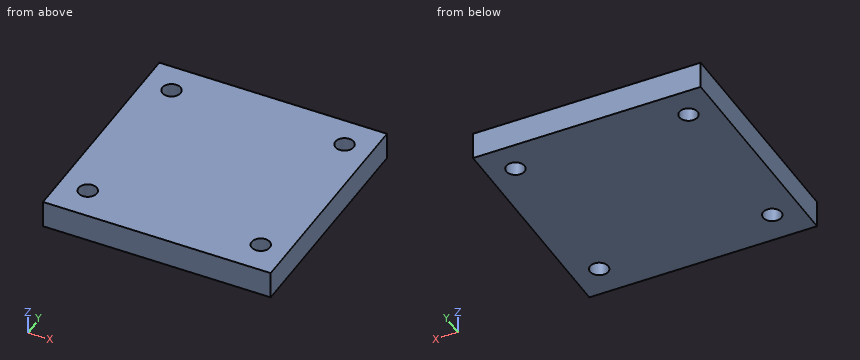
```python
from build123d import *

# Parameters (mm, degrees)
ESQUISSE1_W        = 25
ESQUISSE1_H        = 25
ESQUISSE1_R        = 1
BOSS_EXTRU_1_DEPTH = 3


with BuildPart() as part:
    # Esquisse1 → Boss.-Extru.1 (new body)
    with BuildSketch(Plane.XY):
        with Locations((-1.315129748, -0.313430953)):
            Rectangle(ESQUISSE1_W, ESQUISSE1_H)
        with Locations(Location((-10.74158344, -9.209614493, 0), (0, 0, 180))):
            Circle(ESQUISSE1_R, mode=Mode.SUBTRACT)
        with Locations(Location((-10.74158344, 8.790385507, 0), (0, 0, 180))):
            Circle(ESQUISSE1_R, mode=Mode.SUBTRACT)
        with Locations(Location((8.25841656, -9.209614493, 0), (0, 0, 180))):
            Circle(ESQUISSE1_R, mode=Mode.SUBTRACT)
        with Locations(Location((8.25841656, 8.790385507, 0), (0, 0, 180))):
            Circle(ESQUISSE1_R, mode=Mode.SUBTRACT)
    extrude(amount=BOSS_EXTRU_1_DEPTH)


solid = part.part
```
Work out the finished part from the listing and answer in its coordinate system (mm). Give positions to 0.01 mm unless a question says otherwise; leave off trailing zeros. Write each loop counter-clockwise with the first axis right and the second up, starting at its lowest first coordinate (ties: lowest second). Pieces come first, ordered by that corner, then holes. Notation, with made-up numbers: (-15, 9) -> (44, 9) arc R20 ccw to (44, 18) -> close; hole circle Ø9 at (-12.5, 87). An arc over 180 degrees is marked (long way). Write item = value, one per line.
Q1. Section B-B on y = -9.5 is taken. Determine the outline of the cut face in (x, z), and give its area (3 significant figures).
Computed values:
outline = (-13.82, 0) -> (-11.7, 0) -> (-11.7, 3) -> (-13.82, 3) -> close; (-9.78, 0) -> (7.3, 0) -> (7.3, 3) -> (-9.78, 3) -> close; (9.22, 0) -> (11.18, 0) -> (11.18, 3) -> (9.22, 3) -> close
area = 63.5 mm^2
Q2. Flat-ended cylindrical pins translate along their axes: pin 1 Ø2.5 at (x, y) = (8.26, -9.21) entering from -Z; pin 2 Ø1.2 at (x, y) = (-10.74, -9.21) entering from -Z. Find the tip coordinate at first contact, or state that the pin passes through.
Computed values:
pin_1 = 0
pin_2 = through
Q3. Section A-A on x = 8.75 is taken. Determine the outline of the cut face in (y, z), and give its area (4 significant figures).
Computed values:
outline = (-12.81, 0) -> (-10.08, 0) -> (-10.08, 3) -> (-12.81, 3) -> close; (-8.34, 0) -> (7.92, 0) -> (7.92, 3) -> (-8.34, 3) -> close; (9.66, 0) -> (12.19, 0) -> (12.19, 3) -> (9.66, 3) -> close
area = 64.55 mm^2
Q4. Section C-C on z = 1.3 is taken. Determine the outline of the cut face in (x, y), and give its area (3 significant figures).
Computed values:
outline = (-13.82, -12.81) -> (11.18, -12.81) -> (11.18, 12.19) -> (-13.82, 12.19) -> close; hole circle Ø2 at (-10.74, -9.21); hole circle Ø2 at (-10.74, 8.79); hole circle Ø2 at (8.26, -9.21); hole circle Ø2 at (8.26, 8.79)
area = 612 mm^2
Q5. Consider line 1 along X through (y, z) = (-8.75, 2.35); line 2 along Y through (x, z) = (-10.5, 0.35); line 3 along Y through (x, z) = (-10, 0.95). Determine where each line is inside the solid, lowest interval first.
Computed values:
line_1 = -13.82 to -11.63, -9.85 to 7.37, 9.15 to 11.18
line_2 = -12.81 to -10.18, -8.24 to 7.82, 9.76 to 12.19
line_3 = -12.81 to -9.88, -8.54 to 8.12, 9.46 to 12.19
